from build123d import *

# Parameters (mm, degrees)
F0_R     = 33.85
F1_DEPTH = 20
F2_R     = 33.1
F3_DEPTH = 19
F4_R     = 5
F5_R     = 2.5


with BuildPart() as f1:
    # F0 (on Top) → F1 (new body)
    with BuildSketch(Plane.XY):
        Circle(F0_R)
    extrude(amount=F1_DEPTH)

    # F2 (on face) → F3 (cut)
    with BuildSketch(Plane.XY.offset(20)):
        Circle(F2_R)
    extrude(amount=-F3_DEPTH, mode=Mode.SUBTRACT)

    # F4
    f4_edges = [f1.edges().sort_by_distance(p)[0] for p in [
        (-33.1, 0, 1),
    ]]
    fillet(f4_edges, radius=F4_R)

    # F5
    f5_edges = [f1.edges().sort_by_distance(p)[0] for p in [
        (-33.85, 0, 0),
    ]]
    fillet(f5_edges, radius=F5_R)


solid = f1.part
Verification items for the finished model (mm, model axes). A direction names the side the tool comes from. Give positions to 0.01 mm unless a question says otherwise; leave off trailing zeros. Loops run counter-clockwise (first coordinate to the right, second up) from the corner with the lowest first, then second, coordinate; pieces in that order, holes last.
1) Depth check by flat-ended pin: pin 1 Ø4 at (y, z) = (-11.5, 4) entering from -X; pin 2 Ø12 at (x, y) = (4.5, 23.5) entering from +Z; pin 3 Ø17 at (x, y) = (11.5, 1.5) entering from +Z. Enter the tip coordinate at first touch or a pass-through.
2) Thickness scan on line 1 along Y through (x, z) = (0, 10.5); line 2 along Z through (x, y) = (2, 20.5); line 3 along X through (y, z) = (-24, 13). Record the ranges inside material, lowest first.
3) Draft check along Y on faces 3 (the cylindrical face through (-7.18, -32.31, 13.1)), 4 (the flat face through (7.36, -32.44, 20)), 5 (the cylindrical face through (32.287, 10.168, 11.128)). Enter one of: pulls with the +Y half, pulls with the -Y half, needs draft (parallel to the pull), parting line crosses it, or undercut.
4) Sectioned sample at A-A, the plane x = 0. Enter the section's corners in (y, z).
5) Set-up check for faces 1 (the flat face through (0, 0, 0)), 2 (the flat face through (0, 0, 1)): record each of +Z, -Z, +X, -X, +Y, -Y from which the full face is reachable in a straight line by a thin tool's end or side.
6) Sectioned sample at C-C, the plane z = 10. Enter the section's corners in (x, y), then the cut area to 3 significant figures.
Answers:
1. pin 1: stops at x = -32.49
1. pin 2: stops at z = 1.35
1. pin 3: stops at z = 1
2. line 1: y = -33.85 to -33.1, 33.1 to 33.85
2. line 2: z = 0 to 1
2. line 3: x = -23.87 to -22.79, 22.79 to 23.87
3. face 3: undercut
3. face 4: needs draft
3. face 5: parting line crosses it
4. outline: (-33.85, 2.5) arc R2.5 ccw to (-31.35, 0) - (31.35, 0) arc R2.5 ccw to (33.85, 2.5) - (33.85, 20) - (33.1, 20) - (33.1, 6) arc R5 cw to (28.1, 1) - (-28.1, 1) arc R5 cw to (-33.1, 6) - (-33.1, 20) - (-33.85, 20) - close
5. face 1: -Z, +X, -X, +Y, -Y
5. face 2: +Z
6. outline: circle Ø67.7 at (0, 0); hole circle Ø66.2 at (0, 0)
6. area: 158 mm2
